Here's how the part is built. I have some questions about the finished solid (model axes, mm). A direction names the side the tool comes from. Give positions to 0.01 mm unless a question says otherwise; leave off trailing zeros. Loops run counter-clockwise (first coordinate to the right, second up) from the corner with the lowest first, then second, coordinate; pieces in that order, holes last. Notation, with made-up numbers: (88, -18) - (113, -18) arc R33 cw to (113, 15) - close; hole circle Ø8 at (60, 11). An arc over 180 degrees is marked (long way). Use one line per item in the form item = value.
from build123d import *

# Parameters (mm, degrees)
PAD_DEPTH       = 25
SKETCH001_R     = 4.3
POCKET_DEPTH    = 18.001
SKETCH002_R     = 3.3
POCKET001_DEPTH = 18.001
FILLET_R        = 4
FILLET001_R     = 2
SKETCH003_R     = 6.75
POCKET002_DEPTH = 5
SKETCH005_R     = 5.25
POCKET004_DEPTH = 5


with BuildPart() as part:
    # Sketch → Pad (new body)
    with BuildSketch(Plane.XZ):
        Polygon((72.5, 30.4), (-72.5, 30.4), (-72.5, 20.4), (-39.6, 20.4), (-30, 12.4), (-17.4, 12.4), (-17.4, 22.9), (17.4, 22.9), (17.4, 12.4), (30, 12.4), (39.6, 20.4), (72.5, 20.4), align=None)
    extrude(amount=PAD_DEPTH)

    # Sketch001 (on Face10 of Pad) → Pocket (cut, through all)
    with BuildSketch(Plane(origin=(0, 0, 30.4), x_dir=(-1, 0, 0), z_dir=(0, 0, 1))):
        with Locations((-60, 12.5)):
            Circle(SKETCH001_R)
        with Locations((60, 12.5)):
            Circle(SKETCH001_R)
    extrude(amount=-POCKET_DEPTH, mode=Mode.SUBTRACT)

    # Sketch002 (on Face15 of Pocket) → Pocket001 (cut, through all)
    with BuildSketch(Plane(origin=(0, 0, 30.4), x_dir=(-1, 0, 0), z_dir=(0, 0, 1))):
        with Locations((-23, 6)):
            Circle(SKETCH002_R)
        with Locations((-23, 19)):
            Circle(SKETCH002_R)
        with Locations((23, 19)):
            Circle(SKETCH002_R)
        with Locations((23, 6)):
            Circle(SKETCH002_R)
    extrude(amount=-POCKET001_DEPTH, mode=Mode.SUBTRACT)

    # Fillet
    fillet_edges = [part.edges().sort_by_distance(p)[0] for p in [
        (-72.5, -25, 25.4),
        (-72.5, 0, 25.4),
        (72.5, -25, 25.4),
        (72.5, 0, 25.4),
    ]]
    fillet(fillet_edges, radius=FILLET_R)

    # Fillet001
    fillet001_edges = [part.edges().sort_by_distance(p)[0] for p in [
        (39.6, -12.5, 20.4),
        (-39.6, -12.5, 20.4),
    ]]
    fillet(fillet001_edges, radius=FILLET001_R)

    # Sketch003 (on Face13 of Fillet001) → Pocket002 (cut)
    with BuildSketch(Plane(origin=(0, 0, 30.4), x_dir=(-1, 0, 0), z_dir=(0, 0, 1))):
        with Locations((-60, 12.5)):
            Circle(SKETCH003_R)
        with Locations((60, 12.5)):
            Circle(SKETCH003_R)
    extrude(amount=-POCKET002_DEPTH, mode=Mode.SUBTRACT)

    # Sketch005 (on Face13 of Pocket002) → Pocket004 (cut)
    with BuildSketch(Plane(origin=(0, 0, 30.4), x_dir=(-1, 0, 0), z_dir=(0, 0, 1))):
        with Locations((-23, 19)):
            Circle(SKETCH005_R)
        with Locations((-23, 6)):
            Circle(SKETCH005_R)
        with Locations((23, 6)):
            Circle(SKETCH005_R)
        with Locations((23, 19)):
            Circle(SKETCH005_R)
    extrude(amount=-POCKET004_DEPTH, mode=Mode.SUBTRACT)


solid = part.part
(1) If we section it at A-A (y = -12.5): Give the number of separate pieces and of enclosed holes in the cut face, plus the area to 3 significant figures.
Geometry says:
separate_pieces = 3
enclosed_holes = 0
area = 1,420 mm²
(2) Thinking about a two-plate mould opening in Y: for faces 4 (the cylindrical face through (19.85, -6.99, 18.99)), 5 (the cylindrical face through (71.359, -23.797, 25.47)), 6 (the flat face through (72.5, -12, 25)), which applies, pulls with the +Y half, pulls with the -Y half, needs draft (parallel to the pull), parting line crosses it, or undercut?
Geometry says:
face_4 = undercut
face_5 = pulls with the -Y half
face_6 = needs draft
(3) If I drill on probe 1 along Y at (x, z) = (-23, 21.5); probe 2 along Y at (x, z) = (-23, 27.7); probe 3 along X at (y, z) = (-18.75, 23.75), over which ranges is the centre line in solid material (lowest first)?
Geometry says:
probe_1 = -25 to -22.3, -15.7 to -9.3, -2.7 to 0
probe_2 = -25 to -24.25, -13.75 to -11.25, -0.75 to 0
probe_3 = -72.5 to -26.29, -19.71 to 19.71, 26.29 to 72.5
(4) For faces 1 (the flat face through (19.6, -17.9, 25.4)), 2 (the flat face through (24, -12, 12.4)), 3 (the flat face through (-17.4, -12, 18)), which set-ups out of +Z, -Z, +X, -X, +Y, -Y let a thin tool reach every point of the face, with its end or its side?
Geometry says:
face_1 = +Z
face_2 = -Z, +X, -X, +Y, -Y
face_3 = -Z, +Y, -Y
(5) If we section it at C-C (z = 28.5): List the corners of the cut face in (x, y) for me, plus the area to 3 significant figures.
Geometry says:
outline = (-72.5, -21) arc R4 ccw to (-68.5, -25) - (68.5, -25) arc R4 ccw to (72.5, -21) - (72.5, -4) arc R4 ccw to (68.5, 0) - (-68.5, 0) arc R4 ccw to (-72.5, -4) - close; hole circle Ø13.5 at (-60, -12.5); hole circle Ø10.5 at (-23, -19); hole circle Ø10.5 at (-23, -6); hole circle Ø10.5 at (23, -19); hole circle Ø10.5 at (23, -6); hole circle Ø13.5 at (60, -12.5)
area = 2,980 mm²
(6) If we section it at D-D (x = 60): List the corners of the cut face in (y, z) for me.
Geometry says:
outline = (-25, 20.4) - (-16.8, 20.4) - (-16.8, 25.4) - (-19.25, 25.4) - (-19.25, 30.4) - (-25, 30.4) - close; (-8.2, 20.4) - (0, 20.4) - (0, 30.4) - (-5.75, 30.4) - (-5.75, 25.4) - (-8.2, 25.4) - close
(7) For P1, Ø1, axis at x = 10.5, y = -19, coming from the -Z side; P2, Ø12.5, axis at x = 56.5, y = -18.5, coming from the -Z side; P3, Ø4, axis at x = 23, y = -19, coming from the -Z side; P4, Ø7, axis at x = 60.5, y = -15, coming from the +Z side, each with a flat end and sliding along its axis, tell me the tip position at first contact or that it passes through.
Geometry says:
P1 = 22.9
P2 = 20.4
P3 = through
P4 = 25.4
(8) If we section it at B-B (x = -23): List the corners of the cut face in (y, z) for me, plus the area to 3 significant figures.
Geometry says:
outline = (-25, 12.4) - (-22.3, 12.4) - (-22.3, 25.4) - (-24.25, 25.4) - (-24.25, 30.4) - (-25, 30.4) - close; (-15.7, 12.4) - (-9.3, 12.4) - (-9.3, 25.4) - (-11.25, 25.4) - (-11.25, 30.4) - (-13.75, 30.4) - (-13.75, 25.4) - (-15.7, 25.4) - close; (-2.7, 12.4) - (0, 12.4) - (0, 30.4) - (-0.75, 30.4) - (-0.75, 25.4) - (-2.7, 25.4) - close
area = 173 mm²
